```python
from build123d import *


with BuildPart() as f1:
    # F0 (on Front) → F1 (revolve)
    with BuildSketch(Plane.XZ):
        Polygon((-111.149055, -272.929926), (8.850945, -272.929926), (8.850945, 107.070074), (7.850945, 107.070074), (7.850945, 93.990135), (7.850945, 77.707144), (7.850945, 53.990135), (7.850945, 37.707144), (7.850945, 13.990135), (7.850945, -2.292856), (7.850945, -26.009865), (7.850945, -42.292856), (7.850945, -66.009865), (7.850945, -82.292856), (7.850945, -106.009865), (7.850945, -122.292856), (7.850945, -146.009865), (7.850945, -162.292856), (7.850945, -262.929926), (6.850945, -262.929926), (-111.149055, -262.929926), align=None)
        Polygon((7.850945, 93.990135), (7.850945, 107.070074), (7.850945, 137.070074), (7.850945, 177.070074), (6.850945, 177.070074), (6.850945, 117.070074), (6.850945, 94.627206), (-8.75799, 87.34864), (-8.75799, 84.34864), (6.850945, 77.070074), (6.850945, 54.627206), (-8.75799, 47.34864), (-8.75799, 44.34864), (6.850945, 37.070074), (6.850945, 14.627206), (-8.75799, 7.34864), (-8.75799, 4.34864), (6.850945, -2.929926), (6.850945, -25.372794), (-8.75799, -32.65136), (-8.75799, -35.65136), (6.850945, -42.929926), (6.850945, -65.372794), (-8.75799, -72.65136), (-8.75799, -75.65136), (6.850945, -82.929926), (6.850945, -105.372794), (-8.75799, -112.65136), (-8.75799, -115.65136), (6.850945, -122.929926), (6.850945, -145.372794), (-8.75799, -152.65136), (-8.75799, -155.65136), (6.850945, -162.929926), (6.850945, -262.929926), (7.850945, -262.929926), (7.850945, -162.292856), (-7.75799, -155.01429), (-7.75799, -153.28843), (7.850945, -146.009865), (7.850945, -122.292856), (-7.75799, -115.01429), (-7.75799, -113.28843), (7.850945, -106.009865), (7.850945, -82.292856), (-7.75799, -75.01429), (-7.75799, -73.28843), (7.850945, -66.009865), (7.850945, -42.292856), (-7.75799, -35.01429), (-7.75799, -33.28843), (7.850945, -26.009865), (7.850945, -2.292856), (-7.75799, 4.98571), (-7.75799, 6.71157), (7.850945, 13.990135), (7.850945, 37.707144), (-7.75799, 44.98571), (-7.75799, 46.71157), (7.850945, 53.990135), (7.850945, 77.707144), (-7.75799, 84.98571), (-7.75799, 86.71157), align=None)
        Polygon((7.850945, 177.070074), (7.850945, 137.070074), (8.850945, 137.070074), (8.850945, 237.070074), (7.850945, 237.070074), (7.850945, 277.070074), (-40.149055, 277.070074), (-40.149055, 237.070074), (-41.149055, 237.070074), (-41.149055, 202.070074), (7.850945, 202.070074), align=None)
        Polygon((7.850945, 77.707144), (7.850945, 93.990135), (-7.75799, 86.71157), (-7.75799, 84.98571), align=None)
        Polygon((7.850945, 37.707144), (7.850945, 53.990135), (-7.75799, 46.71157), (-7.75799, 44.98571), align=None)
        Polygon((7.850945, -2.292856), (7.850945, 13.990135), (-7.75799, 6.71157), (-7.75799, 4.98571), align=None)
        Polygon((7.850945, -42.292856), (7.850945, -26.009865), (-7.75799, -33.28843), (-7.75799, -35.01429), align=None)
        Polygon((-7.75799, -75.01429), (7.850945, -82.292856), (7.850945, -66.009865), (-7.75799, -73.28843), align=None)
        Polygon((-7.75799, -115.01429), (7.850945, -122.292856), (7.850945, -106.009865), (-7.75799, -113.28843), align=None)
        Polygon((-7.75799, -155.01429), (7.850945, -162.292856), (7.850945, -146.009865), (-7.75799, -153.28843), align=None)
    revolve(axis=Axis((358.850945, 0, -351.682112), (0, 0, -1)))


solid = f1.part
```
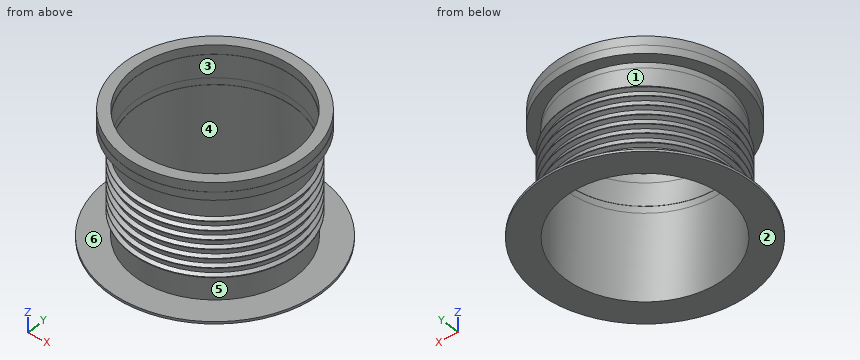
Could you check a few things on this model? Use its own coordinates, in mm. Face numbers are marked on the shaded views. A direction names the side the tool comes from. Coordinates: 2 decimals unless noted, no trailing zeros. Write each loop counter-clockwise with the first axis right and the second up, starting at its lowest first coordinate (ties: lowest second). Pieces come first, ordered by that corner, then holes. Notation, with made-up numbers: (7, 33.25) - (34, 33.25) arc R21 cw to (34, 55.25) - close; hole circle Ø9 at (-18, 75). An arc over 180 degrees is marked (long way). Use a Markdown table: item, result.
Q1. Imagine slicing it at A-A (z = 162). List the corners of the cut face in (x, y) for me, and give its area (3 significant figures).
Geometry check:
| item | result |
|---|---|
| outline | circle Ø704 at (358.85, 0); hole circle Ø700 at (358.85, 0) |
| area | 4,410 mm2 |
Q2. Please list where these lines run through material, in increasing order: L1, parallel to Y at x = 369, z = 186.5; L2, parallel to Z at x = 512, y = 367; L3, parallel to Y at x = 411, z = -190.
Geometry check:
| item | result |
|---|---|
| L1 | y = -350.85 to -349.85, 349.85 to 350.85 |
| L2 | z = -272.93 to -262.93, 202.07 to 277.07 |
| L3 | y = -348.12 to -346.09, 346.09 to 348.12 |
Q3. Thinking about a two-plate mould opening in Y: for the marked faces 3, 4, 5 and 6, which applies, +Y half, -Y half, draft (parallel to the pull), parting line (faces both ways), or undercut?
Geometry check:
| item | result |
|---|---|
| face 3 | undercut |
| face 4 | undercut |
| face 5 | parting line |
| face 6 | draft |
Q4. Which directions (+Z, -Z, +X, -X, +Y, -Y) give clear straight access to the entire face, cutting with the end or side of a thin tool? Please do the marked faces 1 and 2.
Geometry check:
| item | result |
|---|---|
| face 1 | none |
| face 2 | -Z, +X, -X, +Y, -Y |
Q5. I'm going to push flat-ended pins straight in: pin 1 Ø10 at (x, z) = (175, 216) entering from +Y; pin 2 Ø1.5 at (y, z) = (-11.5, -198) entering from -X; pin 3 Ø8 at (y, z) = (246.5, -157.5) entering from +X. Where does each tip first touch, or does it pass through?
Geometry check:
| item | result |
|---|---|
| pin 1 | stops at y = 357.79 |
| pin 2 | stops at x = 7.02 |
| pin 3 | stops at x = 634.73 |
